from build123d import *

# Parameters (mm, degrees)
BOSS_EXTRUDE1_DEPTH = 3.175
SKETCH3_R           = 22.596080088
BOSS_EXTRUDE2_DEPTH = 0.0254
DOME1_FACE_RADIUS   = 22.596080088
DOME1_HEIGHT        = 6.35
SKETCH4_R           = 15.615239036
CUT_EXTRUDE1_DEPTH  = 7.6454


with BuildPart() as part:
    # Sketch1 → Boss-Extrude1 (new body)
    with BuildSketch(Plane.XY):
        with BuildLine():
            add(Edge.make_bspline(
                [(50.828602384, 7910.062180707), (50.828602053, 7901.026169372), (45.984663658, 7892.676550548), (38.121451499, 7888.158544715)],
                knots=[0, 0, 0, 0, 1, 1, 1, 1], degree=3))
            add(Edge.make_bspline(
                [(38.121451499, 7888.158544715), (30.258239339, 7883.640539048), (20.570362548, 7883.640539048), (12.707150389, 7888.158544715)],
                knots=[0, 0, 0, 0, 1, 1, 1, 1], degree=3))
            add(Edge.make_bspline(
                [(12.707150389, 7888.158544715), (4.84393823, 7892.676550548), (-1.66e-07, 7901.026169372), (1.66e-07, 7910.062180707)],
                knots=[0, 0, 0, 0, 1, 1, 1, 1], degree=3))
            add(Edge.make_bspline(
                [(1.66e-07, 7910.062180707), (1.66e-07, 7919.098192041), (4.843938561, 7927.447810866), (12.70715072, 7931.965816533)],
                knots=[0, 0, 0, 0, 1, 1, 1, 1], degree=3))
            add(Edge.make_bspline(
                [(12.70715072, 7931.965816533), (20.570362879, 7936.4838222), (30.25823967, 7936.4838222), (38.12145183, 7931.965816533)],
                knots=[0, 0, 0, 0, 1, 1, 1, 1], degree=3))
            add(Edge.make_bspline(
                [(38.12145183, 7931.965816533), (45.984663989, 7927.447810866), (50.828602384, 7919.098192041), (50.828602384, 7910.062180707)],
                knots=[0, 0, 0, 0, 1, 1, 1, 1], degree=3))
        make_face()
    extrude(amount=BOSS_EXTRUDE1_DEPTH)

    # Sketch3 → Boss-Extrude2 (add)
    with BuildSketch(Plane.XY):
        with Locations((25.414301275, 7910.062180707)):
            Circle(SKETCH3_R)
    extrude(amount=-BOSS_EXTRUDE2_DEPTH)

    # Dome1: a dome of height H over a round flat face of radius A is a cap of a sphere of radius (A * A + H * H) / (2 * H)
    dome1_r = (DOME1_FACE_RADIUS * DOME1_FACE_RADIUS + DOME1_HEIGHT * DOME1_HEIGHT) / (2 * DOME1_HEIGHT)
    dome1_base = Plane((25.414301275, 7910.062180707, -0.0254), z_dir=(0, 0, -1))
    with Locations(dome1_base.offset(DOME1_HEIGHT - dome1_r)):
        dome1_ball = Sphere(dome1_r, mode=Mode.PRIVATE)
    add(split(dome1_ball, bisect_by=dome1_base, keep=Keep.TOP, mode=Mode.PRIVATE))

    # Sketch4 → Cut-Extrude1 (cut)
    with BuildSketch(Plane.XY):
        with Locations((25.409073045, 7919.859985206)):
            Circle(SKETCH4_R)
        with BuildLine():
            Line((28.51760754, 7900.091765684), (28.494324255, 7895.893452368))
            add(Edge.make_bspline(
                [(28.494324255, 7895.893452368), (32.487462639, 7895.777439774), (36.195197067, 7896.275514066), (39.779692278, 7897.341394667)],
                knots=[0, 0, 0, 0, 1, 1, 1, 1], degree=3))
            add(Edge.make_bspline(
                [(39.779692278, 7897.341394667), (42.236438359, 7901.275546963), (43.39540576, 7905.766244587), (42.606935871, 7910.885075863)],
                knots=[0, 0, 0, 0, 1, 1, 1, 1], degree=3))
            add(Edge.make_bspline(
                [(42.606935871, 7910.885075863), (41.151916565, 7907.286794723), (36.579479185, 7902.130368587), (28.51760754, 7900.091765684)],
                knots=[0, 0, 0, 0, 1, 1, 1, 1], degree=3))
        make_face()
        with BuildLine():
            Line((22.24306336, 7900.114149944), (22.266408875, 7895.915841924))
            add(Edge.make_bspline(
                [(22.266408875, 7895.915841924), (18.262512647, 7895.79981609), (14.544790967, 7896.297898327), (10.950640012, 7897.363778928)],
                knots=[0, 0, 0, 0, 1, 1, 1, 1], degree=3))
            add(Edge.make_bspline(
                [(10.950640012, 7897.363778928), (8.487275043, 7901.297931223), (7.408160638, 7905.705876198), (8.198755615, 7910.824707474)],
                knots=[0, 0, 0, 0, 1, 1, 1, 1], degree=3))
            add(Edge.make_bspline(
                [(8.198755615, 7910.824707474), (9.657694086, 7907.226426334), (14.159473448, 7902.152752848), (22.24306336, 7900.114149944)],
                knots=[0, 0, 0, 0, 1, 1, 1, 1], degree=3))
        make_face()
    extrude(amount=-CUT_EXTRUDE1_DEPTH, mode=Mode.SUBTRACT)


solid = part.part
Input: part model. Units: mm. Frame: model coordinates. Give positions to 0.01 mm unless a question says otherwise; leave off trailing zeros. Answer as a JSON object with one key per item and string values. Group by question number.
Item 1: Pin query (flat end, axial travel): P1, Ø2, axis at x = 8, y = 7923.5, coming from the -Z side; P2, Ø7, axis at x = 17, y = 7900.5, coming from the -Z side; P3, Ø25, axis at x = 25.41, y = 7919.86, coming from the -Z side. Return the tip coordinate at first contact, or that it passes through.
Item 2: Cut plane A-A, the plane z = -1.25. State how many separate pieces and enclosed holes the cut face has, and give its area (3 significant figures).
Item 3: Pull-direction query (Y, two-part tool) for faces 1 (the flat face through (26, 7910, 3.175)), 2 (the flat face through (36, 7902, 0)); classes: released by +Y, released by -Y, zero draft, split by the parting line, or undercut.
Item 4: Line query: probe 1 along Z at (x, y) = (18.5, 7921.5) (3 decimals); probe 2 along X at (y, z) = (7917, -0.5); probe 3 along X at (y, z) = (7925, -0.5). Output: solid intervals per line, ascending.
Checks:
{
 "1": {"P1": "stops at z = -0.96", "P2": "stops at z = -5.38", "P3": "stops at z = 0"},
 "2": {"separate pieces": "1", "enclosed holes": "2", "area": "479 mm²"},
 "3": {"face 1": "zero draft", "face 2": "undercut"},
 "4": {"probe 1": "z = 0 to 3.175", "probe 2": "x = 4.75 to 10.06, 40.76 to 46.08", "probe 3": "x = 9.54 to 10.66, 40.15 to 41.29"}
}
